Part print with two shaded views. Sizes in mm from the minimum x, y, z corner. A direction names the side the tool comes from. Round coordinates to 2 decimals unless told otherwise and drop trailing zeros. Loops run counter-clockwise (first coordinate to the right, second up) from the corner with the lowest first, then second, coordinate; pieces in that order, holes last. Notation, with made-up numbers: (-1, 32) - (32, 32) arc R18 cw to (32, 44) - close; hole circle Ø8 at (33.25, -19.5). An arc over 180 degrees is marked (long way). One line per question, with ' | ' between items.
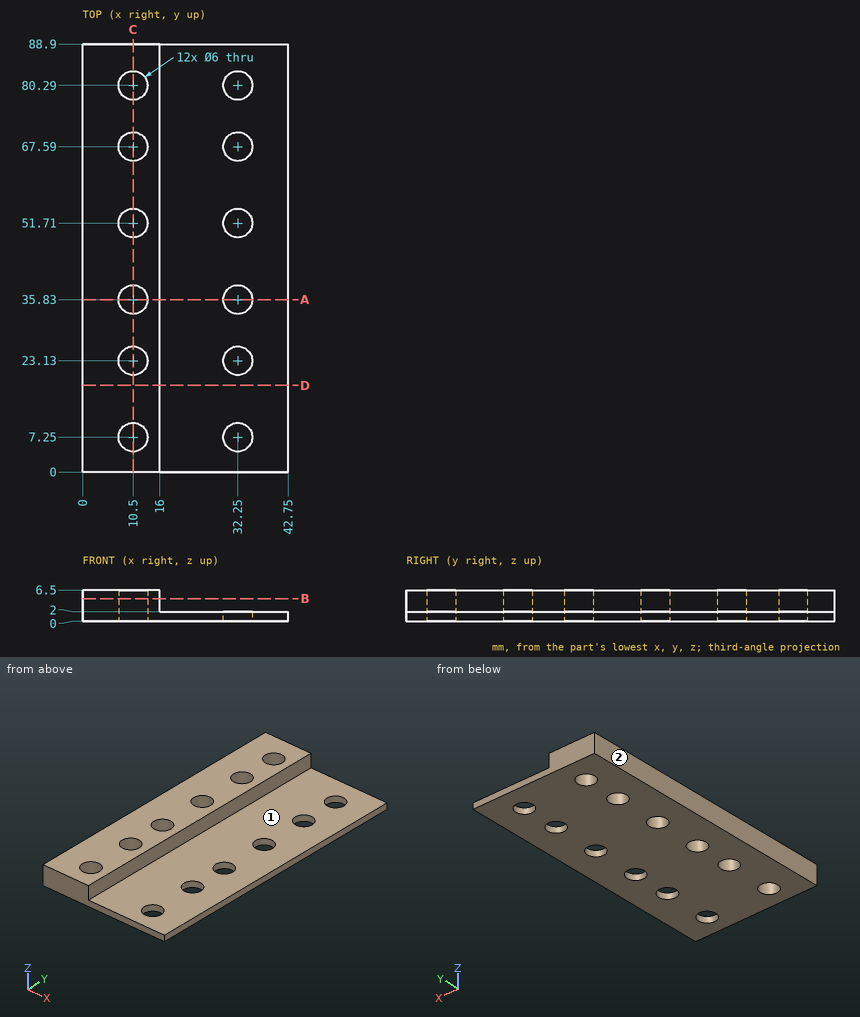
(1) Probe L1, parallel to Z at x = 23.5, y = 63; L2, parallel to X at y = 7, z = 3.75; L3, parallel to X at y = 46, z = 3. List the from-to ranges inside material, lowest first.
Results found:
L1: z = 0 to 2 | L2: x = 0 to 7.51, 13.49 to 16 | L3: x = 0 to 16
(2) Drop flat-ended pins along their axis: P1, Ø9.5, axis at x = 10.5, y = 7.25, coming from the -Z side; P2, Ø9.5, axis at x = 32.25, y = 80.29, coming from the +Z side. Give the stop position or say it passes through.
Results found:
P1: stops at z = 0 | P2: stops at z = 2
(3) Cut at C-C, the plane x = 10.5. Write the cut outline in (y, z), then the cut area to 3 significant figures.
Results found:
outline: (0, 0) - (4.25, 0) - (4.25, 6.5) - (0, 6.5) - close; (10.25, 0) - (20.13, 0) - (20.13, 6.5) - (10.25, 6.5) - close; (26.13, 0) - (32.83, 0) - (32.83, 6.5) - (26.13, 6.5) - close; (38.83, 0) - (48.71, 0) - (48.71, 6.5) - (38.83, 6.5) - close; (54.71, 0) - (64.59, 0) - (64.59, 6.5) - (54.71, 6.5) - close; (70.59, 0) - (77.29, 0) - (77.29, 6.5) - (70.59, 6.5) - close; (83.29, 0) - (88.9, 0) - (88.9, 6.5) - (83.29, 6.5) - close | area: 344 mm²
(4) Tool access for the marked faces 1 and 2: list every direction of +Z, -Z, +X, -X, +Y, -Y with a clear straight run to the whole face (end or side of a thin tool).
Results found:
face 1: +Z, +X, +Y, -Y | face 2: +Z, -Z, -X, +Y, -Y
(5) Cut at D-D, the plane y = 18. Write the cut outline in (x, z).
Results found:
outline: (0, 0) - (42.75, 0) - (42.75, 2) - (16, 2) - (16, 6.5) - (0, 6.5) - close
(6) Cut at A-A, the plane y = 35.83. Write the cut outline in (x, z).
Results found:
outline: (0, 0) - (7.5, 0) - (7.5, 6.5) - (0, 6.5) - close; (13.5, 0) - (29.25, 0) - (29.25, 2) - (16, 2) - (16, 6.5) - (13.5, 6.5) - close; (35.25, 0) - (42.75, 0) - (42.75, 2) - (35.25, 2) - close
(7) Cut at B-B, the plane z = 4.75. Write the cut outline in (x, y), then the cut area to 3 significant figures.
Results found:
outline: (0, 0) - (16, 0) - (16, 88.9) - (0, 88.9) - close; hole circle Ø6 at (10.5, 7.25); hole circle Ø6 at (10.5, 23.13); hole circle Ø6 at (10.5, 35.83); hole circle Ø6 at (10.5, 51.71); hole circle Ø6 at (10.5, 67.59); hole circle Ø6 at (10.5, 80.29) | area: 1,250 mm²
